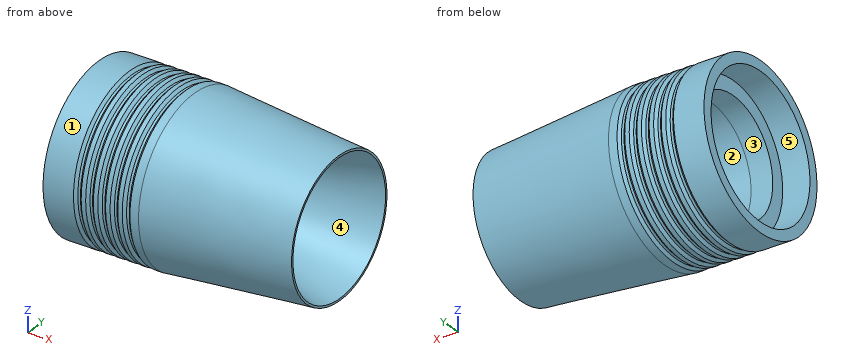
from build123d import *

# Parameters (mm, degrees)
SKETCH4_W       = 29.744523245
SKETCH4_H       = 12.7
SKETCH5_W       = 1.5875
SKETCH5_H       = 1.6129
LPATTERN1_COUNT = 5
LPATTERN1_PITCH = 7.62


with BuildPart() as part:
    # Sketch1 → Revolve1 (revolve)
    with BuildSketch(Plane.XY):
        with BuildLine():
            ThreePointArc((0, 17.653), (0.898160183, 17.712068298), (1.780848569, 17.888255676))
            Line((1.780848569, 17.888255676), (90.17, 41.656))
            Line((90.17, 41.656), (90.17, 42.91114721))
            Line((90.17, 42.91114721), (0, 50.8))
            Line((0, 50.8), (-59.69, 50.8))
            Line((-59.69, 50.8), (-59.69, 44.45))
            Line((-59.69, 44.45), (-72.39, 44.45))
            Line((-72.39, 44.45), (-72.39, 38.1))
            Line((-72.39, 38.1), (-59.69, 38.1))
            Line((-59.69, 38.1), (-9.310840107, 19.331058169))
            ThreePointArc((-9.310840107, 19.331058169), (-4.730423414, 18.075866931), (0, 17.653))
        make_face()
    revolve(axis=Axis((0, 0, 0), (-1, 0, 0)))

    # Sketch2 → Cut-Revolve2 (revolve, cut)
    with BuildSketch(Plane.XY):
        Polygon((25.4, 31.75), (0, 31.75), (-42.645476755, 31.75), (-50.8, 31.75), (-50.8, 0), (0, 0), (25.4, 0), align=None)
        Polygon((-42.645476755, 31.75), (0, 31.75), (25.4, 31.75), (-29.085538438, 35.56), (-42.645476755, 35.56), align=None)
    revolve(axis=Axis((-50.8, 0, 0), (1, 0, 0)), mode=Mode.SUBTRACT)

    # Sketch4 → Cut-Revolve4 (revolve, cut)
    with BuildSketch(Plane.XY):
        with Locations((-57.517738378, 38.1)):
            Rectangle(SKETCH4_W, SKETCH4_H)
    revolve(axis=Axis((0, 0, 0), (-1, 0, 0)), mode=Mode.SUBTRACT)

    # Sketch5 → Cut-Revolve5 (revolve, cut)
    with BuildSketch(Plane.XY):
        Polygon((-37.4396, 50.8), (-37.4396, 49.1871), (-35.8267, 50.8), align=None)
        with Locations((-38.23335, 49.99355)):
            Rectangle(SKETCH5_W, SKETCH5_H)
        Polygon((-40.64, 50.8), (-39.0271, 49.1871), (-39.0271, 50.8), align=None)
    cut_revolve5 = revolve(axis=Axis((0, 0, 0), (-1, 0, 0)), mode=Mode.SUBTRACT)

    # LPattern1: Cut-Revolve5 ×5
    with Locations(*[(i * LPATTERN1_PITCH, 0, 0) for i in range(1, LPATTERN1_COUNT)]):
        add(cut_revolve5, mode=Mode.SUBTRACT)


solid = part.part
The model under review builds one solid part; all positions refer to its coordinate system, in mm. Face numbers are marked on the shaded views. A direction names the side the tool comes from. Round coordinates to 2 decimals unless told otherwise and drop trailing zeros. Order: outer loops, then holes, each group sorted by start corner. A loop starts at its lowest first (then second) coordinate and runs counter-clockwise, first axis right, second up. Notation, with made-up numbers: (-9.5, 75) - (33.5, 75) arc R33 cw to (33.5, 108) - close; hole circle Ø3 at (16, 12). An arc over 180 degrees is marked (long way). Use one line per item in the form item = value.
Q1. To check wall thickness, follow line 1 (Z direction, x = -54.25, y = 0); line 2 (Z direction, x = -34, y = 0); line 3 (Y direction, x = 7, z = 16). State the ranges of each line that lie inside material, in increasing order.
Response values:
line_1 = -50.8 to -44.45, 44.45 to 50.8
line_2 = -50.8 to -35.56, 35.56 to 50.8
line_3 = -47.57 to -28.9, 28.9 to 47.57
Q2. Tool access review of the marked faces 4 and 5: name each direction out of +Z, -Z, +X, -X, +Y, -Y from which nothing blocks a thin tool from reaching the whole face with its end or side.
Response values:
face_4 = +X
face_5 = -X
Q3. Mouldability with a two-part tool opening along Y and no side actions: class the marked faces 1, 2 and 3 as pulls with the +Y half, pulls with the -Y half, needs draft (parallel to the pull), parting line crosses it, or undercut.
Response values:
face_1 = parting line crosses it
face_2 = undercut
face_3 = undercut
Q4. Add section A-A on x = 8. Give the boundary of the cut face in (y, z).
Response values:
outline = circle Ø100.2 at (0, 0); hole circle Ø65.93 at (0, 0)
Q5. Add section B-B on x = 80.5. Give the boundary of the cut face in (y, z).
Response values:
outline = circle Ø87.51 at (0, 0); hole circle Ø78.11 at (0, 0)
Q6. Clearance check with flat-ended pins moving along their axes: P1, Ø4, axis at x = 46.5, z = -13.5, coming from the -Y side; P2, Ø5, axis at x = 5.5, z = 16.5, coming from the +Y side; P3, Ø6, axis at x = 36, y = 27.5, coming from the -Z side. State where each tip first meets the part, or that it passes through.
Response values:
P1 = -45.33
P2 = 48.37
P3 = -40.9
